Read the model definition and answer for the solid it produces. Units are mm, in the model's axes. A direction names the side the tool comes from. Give positions to 0.01 mm unless a question says otherwise; leave off trailing zeros. Loops run counter-clockwise (first coordinate to the right, second up) from the corner with the lowest first, then second, coordinate; pieces in that order, holes last. Notation, with made-up numbers: (4, 71) - (60, 71) arc R19 cw to (60, 75) - close; hole circle Ø5 at (-38, -12.5). An arc over 180 degrees is marked (long way). Write item = value, one per line.
```python
from build123d import *

# Parameters (mm, degrees)
SKETCH1_R             = 36.55
SKETCH1_R_2           = 19
EXTRUDE1_DEPTH        = 40
SKETCH2_R             = 34.75
SKETCH2_R_2           = 27.7
EXTRUDE2_DEPTH        = 1
SKETCH3_R             = 34.75
SKETCH3_R_2           = 27.7
EXTRUDE3_DEPTH        = 1
FILLET1_R             = 4
CHAMFER1_SIZE         = 0.5
CHAMFER1_SIZE2        = 1.866025404
CHAMFER1_PART_2_SIZE  = 0.5
CHAMFER1_PART_2_SIZE2 = 1.866025404


with BuildPart() as part:
    # Sketch1 → Extrude1 (new body)
    with BuildSketch(Plane.XY):
        Circle(SKETCH1_R)
        Circle(SKETCH1_R_2, mode=Mode.SUBTRACT)
    extrude(amount=EXTRUDE1_DEPTH)

    # Sketch2 → Extrude2 (cut)
    with BuildSketch(Plane.XY.offset(40)):
        Circle(SKETCH2_R)
        Circle(SKETCH2_R_2, mode=Mode.SUBTRACT)
    extrude(amount=-EXTRUDE2_DEPTH, mode=Mode.SUBTRACT)

    # Sketch3 → Extrude3 (cut)
    with BuildSketch(Plane(origin=(0, 0, 0), x_dir=(-1, 0, 0), z_dir=(0, 0, -1))):
        Circle(SKETCH3_R)
        Circle(SKETCH3_R_2, mode=Mode.SUBTRACT)
    extrude(amount=-EXTRUDE3_DEPTH, mode=Mode.SUBTRACT)

    # Fillet1
    fillet1_edges = [part.edges().sort_by_distance(p)[0] for p in [
        (-19, 0, 0),
        (-19, 0, 40),
    ]]
    fillet(fillet1_edges, radius=FILLET1_R)

    # Chamfer1
    chamfer1_edges = [part.edges().sort_by_distance(p)[0] for p in [
        (-36.55, 0, 0),
    ]]
    chamfer1_side = [part.faces().sort_by_distance(p)[0] for p in [
        (-35.516209886, 0, 0),
    ]]
    chamfer(chamfer1_edges, length=CHAMFER1_SIZE, length2=CHAMFER1_SIZE2, reference=chamfer1_side[0])

    # Chamfer1 part 2
    chamfer1_part_2_edges = [part.edges().sort_by_distance(p)[0] for p in [
        (-36.55, 0, 40),
    ]]
    chamfer1_part_2_side = [part.faces().sort_by_distance(p)[0] for p in [
        (-35.516209886, 0, 40),
    ]]
    chamfer(chamfer1_part_2_edges, length=CHAMFER1_PART_2_SIZE, length2=CHAMFER1_PART_2_SIZE2, reference=chamfer1_part_2_side[0])


solid = part.part
```
1) A cutting plane is placed at C-C on z = 11.5. Determine the outline of the cut face in (x, y), then the cut area to 3 significant figures.
Output:
outline = circle Ø73.1 at (0, 0); hole circle Ø38 at (0, 0)
area = 3,060 mm²
2) Each of these flat-tipped pins is pushed along its axis until it touches: P1, Ø10, axis at x = 26, z = 32.5, coming from the -Y side; P2, Ø23, axis at x = 0, y = 0, coming from the +Z side; P3, Ø3, axis at y = -28, z = 21.5, coming from the -X side; P4, Ø3, axis at x = -13.5, z = 24.5, coming from the -Y side. Where does it stop, or does it pass through?
Output:
P1 = -29.91
P2 = through
P3 = -25.17
P4 = -34.52
3) A tool of negligible diameter and unlimited length cuts with its end or side. For faces 1 (the face through (-23.3, -15.3, 39)), 2 (the face through (-30, 19, 0)), 3 (the face through (-26.42, 8.32, 0.49)), from which of +Z, -Z, +X, -X, +Y, -Y can it reach the whole face along a straight path? Write none if from no direction.
Output:
face_1 = +Z
face_2 = -Z, +X, -X, +Y, -Y
face_3 = -Z
4) Find the intervals of material crossed by probe 1 along Y at (x, z) = (0, 11.5); probe 2 along Y at (x, z) = (0, 39.25); probe 3 along Z at (x, y) = (26, 14), in increasing order.
Output:
probe_1 = -36.55 to -19, 19 to 36.55
probe_2 = -36.25 to -34.75, -27.7 to -20.67, 20.67 to 27.7, 34.75 to 36.25
probe_3 = 1 to 39
5) The mould has two halves that part along X. Classify faces 4 (the face through (-30, 19, 40)), 5 (the face through (-7.92, -35.68, 19.75)), 6 (the face through (18.68, 29.3, 39.51)): pulls with the +X half, pulls with the -X half, needs draft (parallel to the pull), parting line crosses it, or undercut.
Output:
face_4 = needs draft
face_5 = parting line crosses it
face_6 = undercut
